from build123d import *

# Parameters (mm, degrees)
SKETCH1_W               = 44
SKETCH1_H               = 32
BOSS_EXTRUDE1_DEPTH     = 11
SKETCH2_W               = 24.5
SKETCH2_H               = 15.5
CUT_EXTRUDE1_DEPTH      = 7.75
FILLET1_R               = 7.75
CUT_EXTRUDE2_DEPTH      = 40.370833113
CUT_EXTRUDE2_DEPTH_BACK = 40.370833113
SKETCH4_R               = 3
SKETCH4_W               = 20
SKETCH4_H               = 10.5
CUT_EXTRUDE3_DEPTH      = 30.342801502
FILLET4_R               = 5.5
SKETCH7_W               = 10
SKETCH7_H               = 10
SKETCH7_R               = 2
BOSS_EXTRUDE5_DEPTH     = 6
FILLET5_R               = 5
CUT_EXTRUDE7_START      = -3
SKETCH9_R               = 3
SKETCH9_R_2             = 2
CUT_EXTRUDE7_DEPTH      = 3
SKETCH10_R              = 3
CUT_EXTRUDE8_DEPTH      = 4
FILLET7_R               = 10.5
FILLET8_R               = 11


# Some blends are built 0.0001 mm under size
with BuildPart() as part:
    # Sketch1 → Boss-Extrude1 (new body)
    with BuildSketch(Plane(origin=(0, 0, 0), x_dir=(0, 0, -1), z_dir=(1, 0, 0))):
        Rectangle(SKETCH1_W, SKETCH1_H)
    extrude(amount=BOSS_EXTRUDE1_DEPTH)

    # Sketch2 → Cut-Extrude1 (cut)
    with BuildSketch(Plane(origin=(0, 0, 0), x_dir=(0, 0, -1), z_dir=(1, 0, 0))):
        with Locations((0, -5.25)):
            Rectangle(SKETCH2_W, SKETCH2_H)
    extrude(amount=CUT_EXTRUDE1_DEPTH, mode=Mode.SUBTRACT)

    # Fillet1
    fillet1_edges = [part.edges().sort_by_distance(p)[0] for p in [
        (7.75, 2.5, 0),
        (7.75, -13, 0),
    ]]
    fillet(fillet1_edges, radius=FILLET1_R - 0.0001)  # a hair under: the kernel refuses the full size

    # Sketch3 → Cut-Extrude2 (cut, two sides: drawn at the far end of the back side and taken through both)
    with BuildSketch(Plane.XY.offset(-12.25).offset(-CUT_EXTRUDE2_DEPTH_BACK)):
        with BuildLine():
            ThreePointArc((0, -10.25), (3.535533906, -8.785533906), (5, -5.25))
            ThreePointArc((5, -5.25), (3.535533906, -1.714466094), (0, -0.25))
            Line((0, -0.25), (0, -10.25))
        make_face()
        with BuildLine():
            Line((0, -10.25), (0, -0.25))
            ThreePointArc((0, -0.25), (-5, -5.25), (0, -10.25))
        make_face()
    extrude(amount=CUT_EXTRUDE2_DEPTH + CUT_EXTRUDE2_DEPTH_BACK, mode=Mode.SUBTRACT)

    # Sketch4 → Cut-Extrude3 (cut, through all)
    with BuildSketch(Plane(origin=(11, 0, 0), x_dir=(0, 0, -1), z_dir=(1, 0, 0))):
        with Locations((-16, 10)):
            Circle(SKETCH4_R)
        with Locations((16, 10)):
            Circle(SKETCH4_R)
        with Locations((0, 10.75)):
            Rectangle(SKETCH4_W, SKETCH4_H)
    extrude(amount=-CUT_EXTRUDE3_DEPTH, mode=Mode.SUBTRACT)

    # Fillet4
    fillet4_edges = [part.edges().sort_by_distance(p)[0] for p in [
        (5.5, 16, 22),
        (5.5, 16, -22),
    ]]
    fillet(fillet4_edges, radius=FILLET4_R)

    # Sketch7 → Boss-Extrude5 (add)
    with BuildSketch(Plane(origin=(0, 0, 0), x_dir=(0, 0, -1), z_dir=(1, 0, 0))):
        with Locations((0, -21)):
            Rectangle(SKETCH7_W, SKETCH7_H)
        with Locations((0, -21)):
            Circle(SKETCH7_R, mode=Mode.SUBTRACT)
    extrude(amount=BOSS_EXTRUDE5_DEPTH)

    # Fillet5
    fillet5_edges = [part.edges().sort_by_distance(p)[0] for p in [
        (3, -26, -5),
        (3, -26, 5),
    ]]
    fillet(fillet5_edges, radius=FILLET5_R - 0.0001)  # a hair under: the kernel refuses the full size

    # Sketch9 → Cut-Extrude7 (cut)
    with BuildSketch(Plane(origin=(6, 0, 0), x_dir=(0, 0, -1), z_dir=(1, 0, 0)).offset(CUT_EXTRUDE7_START)):
        with Locations((0, -21)):
            Circle(SKETCH9_R)
        with Locations((0, -21)):
            Circle(SKETCH9_R_2, mode=Mode.SUBTRACT)
    extrude(amount=CUT_EXTRUDE7_DEPTH, mode=Mode.SUBTRACT)

    # Sketch10 → Cut-Extrude8 (cut)
    # profile 1 of 2: a face of its own
    with BuildSketch(Plane(origin=(11, 0, 0), x_dir=(0, 0, -1), z_dir=(1, 0, 0))):
        Polygon((-16, 5.381197846), (-12, 7.690598923), (-12, 12.309401077), (-16, 14.618802154), (-20, 12.309401077), (-20, 7.690598923), align=None)
        with Locations((-16, 10)):
            Circle(SKETCH10_R, mode=Mode.SUBTRACT)
    # profile 2 of 2: a face of its own
    with BuildSketch(Plane(origin=(11, 0, 0), x_dir=(0, 0, -1), z_dir=(1, 0, 0))):
        Polygon((16, 5.381197846), (20, 7.690598923), (20, 12.309401077), (16, 14.618802154), (12, 12.309401077), (12, 7.690598923), align=None)
        with Locations((16, 10)):
            Circle(SKETCH10_R, mode=Mode.SUBTRACT)
    extrude(amount=-CUT_EXTRUDE8_DEPTH, mode=Mode.SUBTRACT)

    # Fillet7
    fillet7_edges = [part.edges().sort_by_distance(p)[0] for p in [
        (11, 5.5, 0),
    ]]
    fillet(fillet7_edges, radius=FILLET7_R)

    # Fillet8
    # the kernel refuses this fillet: 11 mm, written as the material it takes off along each edge
    with BuildSketch(Plane(origin=(11, -16, 49.5), x_dir=(0, 1, 0), z_dir=(0, 0, -1))) as fillet8_piece_1_section:
        with BuildLine():
            CenterArc((FILLET8_R, -FILLET8_R), FILLET8_R, 90, 90)
            Line((0, -FILLET8_R), (0, 0))
            Line((0, 0), (FILLET8_R, 0))
        make_face()
    fillet8_piece_1 = extrude(amount=99, mode=Mode.PRIVATE)
    fillet8_piece_1 = split(fillet8_piece_1, bisect_by=Plane(origin=(6, -13.119412113, 27.25), z_dir=(1, 0, 0)), keep=Keep.TOP, mode=Mode.PRIVATE)
    fillet8_piece_1 = split(fillet8_piece_1, bisect_by=Plane(origin=(9.313036117, -13.119412113, 5), z_dir=(0, 0, 1)), keep=Keep.TOP, mode=Mode.PRIVATE)
    add(fillet8_piece_1, mode=Mode.SUBTRACT)
    with BuildSketch(Plane(origin=(11, -16, 49.5), x_dir=(0, 1, 0), z_dir=(0, 0, -1))) as fillet8_piece_2_section:
        with BuildLine():
            CenterArc((FILLET8_R, -FILLET8_R), FILLET8_R, 90, 90)
            Line((0, -FILLET8_R), (0, 0))
            Line((0, 0), (FILLET8_R, 0))
        make_face()
    fillet8_piece_2 = extrude(amount=99, mode=Mode.PRIVATE)
    fillet8_piece_2 = split(fillet8_piece_2, bisect_by=Plane(origin=(6, -15.650616863, 27.25), z_dir=(-1, 0, 0)), keep=Keep.TOP, mode=Mode.PRIVATE)
    fillet8_piece_2 = split(fillet8_piece_2, bisect_by=Plane(origin=(4.102097244, -15.650616863, 5), z_dir=(0, 0, 1)), keep=Keep.TOP, mode=Mode.PRIVATE)
    add(fillet8_piece_2, mode=Mode.SUBTRACT)
    with BuildSketch(Plane(origin=(11, -16, 49.5), x_dir=(0, 1, 0), z_dir=(0, 0, -1))) as fillet8_piece_3_section:
        with BuildLine():
            CenterArc((FILLET8_R, -FILLET8_R), FILLET8_R, 90, 90)
            Line((0, -FILLET8_R), (0, 0))
            Line((0, 0), (FILLET8_R, 0))
        make_face()
    fillet8_piece_3 = extrude(amount=99, mode=Mode.PRIVATE)
    fillet8_piece_3 = split(fillet8_piece_3, bisect_by=Plane(origin=(6, -13.119412113, 0), z_dir=(1, 0, 0)), keep=Keep.TOP, mode=Mode.PRIVATE)
    fillet8_piece_3 = split(fillet8_piece_3, bisect_by=Plane(origin=(9.313036117, -13.119412113, -5), z_dir=(0, 0, 1)), keep=Keep.TOP, mode=Mode.PRIVATE)
    fillet8_piece_3 = split(fillet8_piece_3, bisect_by=Plane(origin=(9.313036117, -13.119412113, 5), z_dir=(0, 0, -1)), keep=Keep.TOP, mode=Mode.PRIVATE)
    add(fillet8_piece_3, mode=Mode.SUBTRACT)
    with BuildSketch(Plane(origin=(11, -16, 49.5), x_dir=(0, 1, 0), z_dir=(0, 0, -1))) as fillet8_piece_4_section:
        with BuildLine():
            CenterArc((FILLET8_R, -FILLET8_R), FILLET8_R, 90, 90)
            Line((0, -FILLET8_R), (0, 0))
            Line((0, 0), (FILLET8_R, 0))
        make_face()
    fillet8_piece_4 = extrude(amount=99, mode=Mode.PRIVATE)
    fillet8_piece_4 = split(fillet8_piece_4, bisect_by=Plane(origin=(6, -13.119412113, -27.25), z_dir=(1, 0, 0)), keep=Keep.TOP, mode=Mode.PRIVATE)
    fillet8_piece_4 = split(fillet8_piece_4, bisect_by=Plane(origin=(9.313036117, -13.119412113, -5), z_dir=(0, 0, -1)), keep=Keep.TOP, mode=Mode.PRIVATE)
    add(fillet8_piece_4, mode=Mode.SUBTRACT)
    with BuildSketch(Plane(origin=(11, -16, 49.5), x_dir=(0, 1, 0), z_dir=(0, 0, -1))) as fillet8_piece_5_section:
        with BuildLine():
            CenterArc((FILLET8_R, -FILLET8_R), FILLET8_R, 90, 90)
            Line((0, -FILLET8_R), (0, 0))
            Line((0, 0), (FILLET8_R, 0))
        make_face()
    fillet8_piece_5 = extrude(amount=99, mode=Mode.PRIVATE)
    fillet8_piece_5 = split(fillet8_piece_5, bisect_by=Plane(origin=(6, -15.650616863, -27.25), z_dir=(-1, 0, 0)), keep=Keep.TOP, mode=Mode.PRIVATE)
    fillet8_piece_5 = split(fillet8_piece_5, bisect_by=Plane(origin=(4.102097244, -15.650616863, -5), z_dir=(0, 0, -1)), keep=Keep.TOP, mode=Mode.PRIVATE)
    add(fillet8_piece_5, mode=Mode.SUBTRACT)


solid = part.part
Model file for the job. Use its own axes, mm. A direction names the side the tool comes from. Coordinates: 2 decimals unless noted, no trailing zeros. Loops run counter-clockwise (first coordinate to the right, second up) from the corner with the lowest first, then second, coordinate; pieces in that order, holes last. Notation, with made-up numbers: (-21.75, 89.5) -> (2.25, 89.5) arc R11 cw to (2.25, 96.5) -> close; hole circle Ø1 at (70, 35.25). An arc over 180 degrees is marked (long way). Use one line per item in the form item = value. Start each with the question number.
(1) Probe probe 1 along Z at (x, y) = (8.25, 10.5); probe 2 along Y at (x, z) = (2.2, 0); probe 3 along Z at (x, y) = (5, 8.5). List the from-to ranges inside material, lowest first. Write a range as from..to.
(2) Pull direction Z, two halves, no side cores. Call faces 6 (the cylindrical face through (3, -24, 4)), 7 (the cylindrical face through (4, 10, 19)), 8 (the flat face through (3, -18, -5)): pulls with the +Z half, pulls with the -Z half, needs draft (parallel to the pull), parting line crosses it, or undercut.
(3) Cut at D-D on y = -15.5. Give the cut face in (x, z).
(4) Tool access for faces 1 (the flat face through (9.028, 13.448, -18.028)), 2 (the cylindrical face through (5.58, 14.35, 20.43)), 3 (the cylindrical face through (7.863, -12.692, 0.308)), 4 (the cylindrical face through (8.01, 2.34, -0.14)), 5 (the flat face through (6, -5, -12.25)): list every direction of +Z, -Z, +X, -X, +Y, -Y with a clear straight run to the whole face (end or side of a thin tool).
(5) Cut at C-C on x = 1.5. Give the number of separate pieces and of enclosed holes in the cut face, and give its area (3 significant figures).
(6) Cut at A-A on y = 10. Give the cut face in (x, z), and give its area (3 significant figures).
(7) Flat gauge pins, fed straight in: pin 1 (3.5 mm diameter, centred on y = 10, z = -16, fed in from -X); pin 2 (5 mm diameter, centred on y = -21.5, z = 1, fed in from +X); pin 3 (1 mm diameter, centred on x = 5.5, y = -19.5, fed in from +Z); pin 4 (2.5 mm diameter, centred on y = 8, z = -14.5, fed in from +X). Where does each tip first touch, or does it go through?
(8) Cut at B-B on z = -15. Give the cut face in (x, y).
Values:
q1.probe_1 = -22..-20, -12..-10, 10..12, 20..22
q1.probe_2 = -26..-23, -19..-12.68, 2.18..5.36
q1.probe_3 = -22..-18.6, -13.4..-10, 10..13.4, 18.6..22
q2.face_6 = pulls with the +Z half
q2.face_7 = undercut
q2.face_8 = pulls with the -Z half
q3.outline = (0, -22) -> (3.28, -22) -> (3.28, -5) -> (6, -5) -> (6, 5) -> (3.28, 5) -> (3.28, 22) -> (0, 22) -> close
q4.face_1 = +X
q4.face_2 = +Z, +X, -X, +Y
q4.face_3 = +X, -Y
q4.face_4 = +X, +Y
q4.face_5 = -X
q5.separate_pieces = 2
q5.enclosed_holes = 3
q5.area = 642 mm2
q6.outline = (0, -22) -> (11, -22) -> (11, -20) -> (7, -20) -> (7, -19) -> (0, -19) -> close; (0, -13) -> (7, -13) -> (7, -12) -> (11, -12) -> (11, -10) -> (0, -10) -> close; (0, 10) -> (11, 10) -> (11, 12) -> (7, 12) -> (7, 13) -> (0, 13) -> close; (0, 19) -> (7, 19) -> (7, 20) -> (11, 20) -> (11, 22) -> (0, 22) -> close
q6.area = 116 mm2
q7.pin_1 = through
q7.pin_2 = 6
q7.pin_3 = 5
q7.pin_4 = 7
q8.outline = (0, -16) arc R11 ccw to (11, -5) -> (11, 5.96) -> (7, 5.96) -> (7, 7.17) -> (0, 7.17) -> (0, -0.25) arc R5 cw to (0, -10.25) -> close; (0, 12.83) -> (7, 12.83) -> (7, 14.04) -> (11, 14.04) -> (11, 16) -> (0, 16) -> close
